Build history of the part. All positions in model axes, mm. A direction names the side the tool comes from. Give positions to 0.01 mm unless a question says otherwise; leave off trailing zeros. Order: outer loops, then holes, each group sorted by start corner. A loop starts at its lowest first (then second) coordinate and runs counter-clockwise, first axis right, second up. Notation, with made-up numbers: (-3.5, 21) - (52.5, 21) arc R19 cw to (52.5, 30) - close; hole circle Ø3 at (27, 69). An arc over 180 degrees is marked (long way). Use a Markdown table: item, result. Add a question column.
(1) Wall check: line 1 (Y direction, x = 56.25, z = -4); line 2 (X direction, y = 11, z = -9); line 3 (Y direction, x = 45, z = -12). Give the ranges that are in metal, low to high.
(2) Slice it at B-B (x = 16.5). Write the cut outline in (y, z).
(3) Flat gauge pins, fed straight in: pin 1 (3 mm diameter, centred on y = 18, z = -4, fed in from -X); pin 2 (8 mm diameter, centred on x = 12.5, z = -13.5, fed in from -Y); pin 3 (3 mm diameter, centred on y = 25.5, z = -4.5, fed in from +X). Where does each tip first touch, or does it go through?
(4) Which spindle directions (+Z, -Z, +X, -X, +Y, -Y) get a long thin tool onto all of the face, cutting with end or side? Do faces 1 (the face through (11, 8, -18)), 2 (the face through (44.41, 0.57, -0.72)), 3 (the face through (1.68, 1.64, -12.74)). Say none if no direction does.
(5) Slice it at C-C (z = -15.25). Count the separate pieces of the cut face and the enclosed holes in it, then the cut area to 3 significant figures.
(6) Slice it at D-D (x = 27). Write the cut outline in (y, z), then the cut area to 3 significant figures.
(7) Slice it at A-A (y = 13). Write the cut outline in (x, z), then the cut area to 3 significant figures.
(8) Mould opens along X. For faces 4 (the face through (-1.15, 31.1, -11.26)), 5 (the face through (44.36, 31.96, -11.12)), 6 (the face through (2.783, 7, -12)), 7 (the face through (67, 20, -19)) say: +X half, -X half, draft (parallel to the pull), parting line (faces both ways), or undercut.
Solid Edge part; units mm, degrees
sketch "Sketch1" plane through (0, 0, 0) normal (0, 0, 1) x (1, 0, 0)
  line L0 (90, 0) -> (0, 0)
  line L1 (0, 0) -> (0, 30)
  line L2 (0, 30) -> (90, 30)
  line L3 (90, 30) -> (90, 0)
extrude "Protrusion1" add sketch "Sketch1" against normal blind 20
draft "Draft_2" angle 10 neutral plane through (45, 15, 0) normal (0, 0, 1) pull direction (0, 0, 1) face at (75.9, 0, -16.4667) face at (90, 25.3, -16.4667) face at (0, 4.7, -16.4667) face at (14.1, 30, -16.4667)
shell "Thinwall_1" thickness 3 removed faces 1 at (78.3216, 3.0195, -20)
fillet "Round_1" radius 3 16 edges at (45, 0, 0) (91.7633, -1.7633, -10) (90, 15, 0) (45, 27.4827, -3) (45, 30, 0) (91.7633, 31.7633, -10) (-1.7633, 31.7633, -10) (0, 15, 0) (-1.7633, -1.7633, -10) (45, 2.5173, -3) (2.5173, 15, -3) (87.4827, 15, -3) (88.9815, 1.0185, -11.5) (1.0185, 1.0185, -11.5) (1.0185, 28.9815, -11.5) (88.9815, 28.9815, -11.5)
sketch "Sketch2" plane through (0, 0, 0) normal (0, 0, 1) x (1, 0, 0)
  circle A0 centre (45, 20) radius 4
extrude "ExtrudedProtrusion_3" add sketch "Sketch2" against normal blind 20
sketch "Sketch3" plane through (0, 0, 0) normal (0, 0, 1) x (1, 0, 0)
  circle A0 centre (78.75, 20) radius 4
  circle A1 centre (67.5, 20) radius 4
  circle A2 centre (56.25, 20) radius 4
extrude "ExtrudedProtrusion_4" add sketch "Sketch3" against normal blind 20
sketch "Sketch4" plane through (0, 0, 0) normal (0, 0, 1) x (1, 0, 0)
  circle A0 centre (78.75, 20) radius 3.5
  circle A1 centre (67.5, 20) radius 3.5
  circle A2 centre (56.25, 20) radius 3.5
  circle A3 centre (45, 20) radius 3.5
extrude "ExtrudedCutout_3" cut sketch "Sketch4" against normal blind 19
sketch "Sketch5" plane through (0, 0, 0) normal (0, 0, 1) x (1, 0, 0)
  line L0 (2.7826, 11.7647) -> (19.7174, 11.7647)
  line L1 (19.7174, 11.7647) -> (19.7174, 3.2353)
  line L2 (19.7174, 3.2353) -> (2.7826, 3.2353)
  line L3 (2.7826, 3.2353) -> (2.7826, 11.7647)
extrude "ExtrudedProtrusion_5" add sketch "Sketch5" against normal blind 20
sketch "Sketch6" plane through (0, 0, 0) normal (0, 0, 1) x (1, 0, 0)
  line L0 (19, 3.75) -> (19, 11.25)
  line L1 (19, 11.25) -> (3.5, 11.25)
  line L2 (3.5, 11.25) -> (3.5, 3.75)
  line L3 (3.5, 3.75) -> (19, 3.75)
extrude "ExtrudedCutout_4" cut sketch "Sketch6" against normal blind 18
Solution:
| question | item | result |
|---|---|---|
| 1 | line 1 | -0.71 to 2.8, 16 to 16.5, 23.5 to 24, 27.2 to 30.71 |
| 1 | line 2 | -1.59 to 1.46, 2.78 to 3.5, 19 to 19.72, 88.54 to 91.59 |
| 1 | line 3 | -2.12 to 0.93, 16 to 16.5, 23.5 to 24, 29.07 to 32.12 |
| 2 | outline | (-3.53, -20) - (-0.48, -20) - (2.08, -5.48) arc R3 cw to (3.24, -3.6) - (3.24, -20) - (11.76, -20) - (11.76, -3) - (24.97, -3) arc R3 cw to (27.92, -5.48) - (30.48, -20) - (33.53, -20) - (30.44, -2.48) arc R3 ccw to (27.48, 0) - (11.25, 0) - (11.25, -18) - (3.75, -18) - (3.75, 0) - (2.52, 0) arc R3 ccw to (-0.44, -2.48) - close |
| 3 | pin 1 | x = -0.97 |
| 3 | pin 2 | y = -3.09 |
| 3 | pin 3 | x = 91.06 |
| 4 | face 1 | +Z |
| 4 | face 2 | +Z, +X, -X, -Y |
| 4 | face 3 | -Z |
| 5 | separate pieces | 6 |
| 5 | enclosed holes | 6 |
| 5 | area | 835 mm2 |
| 6 | outline | (-3.53, -20) - (-0.48, -20) - (2.08, -5.48) arc R3 cw to (5.03, -3) - (24.97, -3) arc R3 cw to (27.92, -5.48) - (30.48, -20) - (33.53, -20) - (30.44, -2.48) arc R3 ccw to (27.48, 0) - (2.52, 0) arc R3 ccw to (-0.44, -2.48) - close |
| 6 | area | 195 mm2 |
| 7 | outline | (-3.53, -20) - (-0.48, -20) - (2.08, -5.48) arc R3 cw to (5.03, -3) - (84.97, -3) arc R3 cw to (87.92, -5.48) - (90.48, -20) - (93.53, -20) - (90.44, -2.48) arc R3 ccw to (87.48, 0) - (2.52, 0) arc R3 ccw to (-0.44, -2.48) - close |
| 7 | area | 375 mm2 |
| 8 | face 4 | -X half |
| 8 | face 5 | draft |
| 8 | face 6 | undercut |
| 8 | face 7 | undercut |
